from build123d import *

# Parameters (mm, degrees)
F0_R     = 4
F0_R_2   = 2
F1_DEPTH = 1.9
F2_DEPTH = 1.99
F4_R     = 1.99
F5_DEPTH = 28


with BuildPart() as f1:
    # F0 (on Front) → F1 (new body, symmetric)
    with BuildSketch(Plane.XZ):
        Circle(F0_R)
        Circle(F0_R_2, mode=Mode.SUBTRACT)
    extrude(amount=F1_DEPTH, both=True)

    # F0 (on Front) → F2 (join, symmetric)
    with BuildSketch(Plane.XZ):
        Circle(F0_R)
        Circle(F0_R_2, mode=Mode.SUBTRACT)
    extrude(amount=F2_DEPTH, both=True)

    # F4 (on offset) → F5 (join)
    with BuildSketch(Plane.XY.offset(2.2)):
        Circle(F4_R)
    extrude(amount=F5_DEPTH)


solid = f1.part
Check sheet for the modelled part. Datum: model origin and axes. Units: mm. A direction names the side the tool comes from. Round coordinates to 2 decimals unless told otherwise and drop trailing zeros. Order: outer loops, then holes, each group sorted by start corner. A loop starts at its lowest first (then second) coordinate and runs counter-clockwise, first axis right, second up.
Q1. Scan lines: L1, parallel to Z at x = 0, y = 1; L2, parallel to X at y = 0.1, z = 14; L3, parallel to Y at x = 0.75, z = 12. Record each from-to range of solid material in increasing order.
Filled sheet:
L1: z = -4 to -2, 2 to 30.2
L2: x = -1.99 to 1.99
L3: y = -1.84 to 1.84
Q2. Cross-section at A-A, the plane z = 0. Enter the section's corners in (x, y), plus the area to 3 significant figures.
Filled sheet:
outline: (-4, -1.99) - (-2, -1.99) - (-2, 1.99) - (-4, 1.99) - close; (2, -1.99) - (4, -1.99) - (4, 1.99) - (2, 1.99) - close
area: 15.9 mm2
Q3. Draft check along Z on faces 1 (the face through (0, 0, 30.2)), 2 (the face through (-2, -1.99, -1)), 3 (the face through (0, 0, -2)), 4 (the face through (-0.867, -0.028, -3.905)). Enter one of: pulls with the +Z half, pulls with the -Z half, needs draft (parallel to the pull), parting line crosses it, or undercut.
Filled sheet:
face 1: pulls with the +Z half
face 2: needs draft
face 3: undercut
face 4: parting line crosses it
Q4. Cross-section at B-B, the plane y = 0. Enter the section's corners in (x, z).
Filled sheet:
outline: (-1.99, 3.47) arc R4 ccw (long way) to (1.99, 3.47) - (1.99, 30.2) - (-1.99, 30.2) - close; hole circle Ø4 at (0, 0)
Q5. Depth check by flat-ended pin: P1, Ø1.5, axis at y = 1.5, z = 5.5, coming from the -X side; P2, Ø1.5, axis at y = -1, z = 24, coming from the -X side; P3, Ø3, axis at x = -2.5, z = 16, coming from the -Y side. Enter the tip coordinate at first touch or a pass-through.
Filled sheet:
P1: stops at x = -1.84
P2: stops at x = -1.97
P3: stops at y = -1.72
Q6. Set-up check for faces 5 (the face through (-2, 1.99, -1)), 6 (the face through (-0.259, 1.973, 16.648)): record each of +Z, -Z, +X, -X, +Y, -Y from which the full face is reachable in a straight line by a thin tool's end or side.
Filled sheet:
face 5: +Z, -Z, +X, -X, +Y
face 6: +Z
Q7. Cross-section at D-D, the plane z = 14.5. Enter the section's corners in (x, y).
Filled sheet:
outline: circle Ø3.98 at (0, 0)
Q8. Cross-section at C-C, the plane x = 1. Enter the section's corners in (y, z).
Filled sheet:
outline: (-1.99, -3.87) - (1.99, -3.87) - (1.99, -1.73) - (-1.99, -1.73) - close; (-1.99, 1.73) - (1.99, 1.73) - (1.99, 3.87) - (1.72, 3.87) - (1.72, 30.2) - (-1.72, 30.2) - (-1.72, 3.87) - (-1.99, 3.87) - close
